from build123d import *

# Parameters (mm, degrees)
SKIZZE1_W                                           = 135.069444444
SKIZZE1_H                                           = 50
AUFSATZ_LINEAR_AUSTRAGEN1_DEPTH                     = 200
STIRNSENKUNG_F_R_M8_SENKSCHRAUBE_KOPF_B_D           = 9
STIRNSENKUNG_F_R_M8_SENKSCHRAUBE_KOPF_B_CBORE_D     = 15
STIRNSENKUNG_F_R_M8_SENKSCHRAUBE_KOPF_B_CBORE_DEPTH = 34.5
STIRNSENKUNG_F_R_M8_SENKSCHRAUBE_KO_2_D             = 9
STIRNSENKUNG_F_R_M8_SENKSCHRAUBE_KO_2_DEPTH         = 50
STIRNSENKUNG_F_R_M8_SENKSCHRAUBE_KO_2_CBORE_D       = 15
STIRNSENKUNG_F_R_M8_SENKSCHRAUBE_KO_2_CBORE_DEPTH   = 6.5


with BuildPart() as part:
    # Skizze1 → Aufsatz-Linear austragen1 (new body)
    with BuildSketch(Plane.XY):
        Rectangle(SKIZZE1_W, SKIZZE1_H)
    extrude(amount=AUFSATZ_LINEAR_AUSTRAGEN1_DEPTH)

    # Stirnsenkung f_r M8 Senkschraube _Kopf B (through all)
    with Locations(Plane(origin=(0, 25, 0), x_dir=(1, 0, 0), z_dir=(0, 1, 0))):
        with Locations((0, -150)):
            stirnsenkung_f_r_m8_senkschraube_kopf_b = CounterBoreHole(STIRNSENKUNG_F_R_M8_SENKSCHRAUBE_KOPF_B_D / 2, STIRNSENKUNG_F_R_M8_SENKSCHRAUBE_KOPF_B_CBORE_D / 2, STIRNSENKUNG_F_R_M8_SENKSCHRAUBE_KOPF_B_CBORE_DEPTH)

    # Stirnsenkung f_r M8 Senkschraube _Ko 2
    with Locations(Plane(origin=(0, -25, 0), x_dir=(-1, 0, 0), z_dir=(0, -1, 0))):
        with Locations((0, -150)):
            stirnsenkung_f_r_m8_senkschraube_ko_2 = CounterBoreHole(STIRNSENKUNG_F_R_M8_SENKSCHRAUBE_KO_2_D / 2, STIRNSENKUNG_F_R_M8_SENKSCHRAUBE_KO_2_CBORE_D / 2, STIRNSENKUNG_F_R_M8_SENKSCHRAUBE_KO_2_CBORE_DEPTH, depth=STIRNSENKUNG_F_R_M8_SENKSCHRAUBE_KO_2_DEPTH)

    # Spiegeln1: Stirnsenkung f_r M8 Senkschraube _Kopf B, Stirnsenkung f_r M8 Senkschraube _Ko 2 across plane
    add(stirnsenkung_f_r_m8_senkschraube_kopf_b.mirror(Plane.XY.offset(100)), mode=Mode.SUBTRACT)
    add(stirnsenkung_f_r_m8_senkschraube_ko_2.mirror(Plane.XY.offset(100)), mode=Mode.SUBTRACT)

    # Skizze10 → Kernloch für M8 Helicoil1 (revolve, cut)
    with BuildSketch(Plane(origin=(-52.534722222, 25, 185), x_dir=(0, 0, 1), z_dir=(1, 0, 0))):
        Polygon((0, 0), (0, 32.493571569), (4.15, 30), (4.15, 0), align=None)
    kernloch_f_r_m8_helicoil1 = revolve(axis=Axis((-52.534722222, 31.35, 185), (0, -1, 0)), mode=Mode.SUBTRACT)

    # Spiegeln2: Kernloch für M8 Helicoil1 across plane
    add(kernloch_f_r_m8_helicoil1.mirror(Plane(origin=(0, 0, 0), x_dir=(0, 0, 1), z_dir=(1, 0, 0))), mode=Mode.SUBTRACT)

    # Spiegeln3: Kernloch für M8 Helicoil1 across plane
    add(kernloch_f_r_m8_helicoil1.mirror(Plane.XY.offset(100)), mode=Mode.SUBTRACT)

    # Spiegeln3 copy 1 sketch → Spiegeln3 copy 1 (revolve, cut)
    with BuildSketch(Plane(origin=(52.534722222, 25, 15), x_dir=(0, 0, -1), z_dir=(-1, 0, 0))):
        Polygon((0, 0), (0, 32.493571569), (4.15, 30), (4.15, 0), align=None)
    revolve(axis=Axis((52.534722222, 31.35, 15), (0, -1, 0)), mode=Mode.SUBTRACT)


solid = part.part
Model file for the job. Use its own axes, mm. A direction names the side the tool comes from. Coordinates: 2 decimals unless noted, no trailing zeros. Order: outer loops, then holes, each group sorted by start corner. A loop starts at its lowest first (then second) coordinate and runs counter-clockwise, first axis right, second up. Notation, with made-up numbers: (53, 69) -> (102, 69) arc R22 ccw to (102, 89) -> close; hole circle Ø8 at (85.5, 3). An arc over 180 degrees is marked (long way). Return JSON: item names as keys, results as strings. Group by question number.
Item 1: Saw through at B-B on z = 150. Write the cut outline in (x, y).
Item 2: Saw through at C-C on y = 0.5. Write the cut outline in (x, z).
Item 3: Pull direction Z, two halves, no side cores. Call faces 4 (the flat face through (-1, 0, 0)), 5 (the cylindrical face through (0.98, -14.06, 154.39)), 6 (the cylindrical face through (50.01, 10.21, 181.707)), 7 (the flat face through (-1, 0, 200)): pulls with the +Z half, pulls with the -Z half, needs draft (parallel to the pull), parting line crosses it, or undercut.
Item 4: Wall check: line 1 along X through (y, z) = (3.5, 185); line 2 along Z through (x, y) = (0, 12); line 3 along Z through (x, y) = (0, -15.75). Give the ranges that are in metal, low to high. Write a range as [from, to].
Item 5: Tool access for faces 1 (the cylindrical face through (0.976, -21.796, 57.436)), 2 (the flat face through (-1, -25, 99)), 3 (the cylindrical face through (48.483, 10.21, 15.9)): list every direction of +Z, -Z, +X, -X, +Y, -Y with a clear straight run to the whole face (end or side of a thin tool).
Item 6: Flat gauge pins, fed straight in: P1, Ø2, axis at x = 30, y = -13, coming from the -Z side; P2, Ø4.5, axis at x = 2, z = 148.5, coming from the +Y side; P3, Ø7.5, axis at x = 52.53, z = 185, coming from the +Y side; P4, Ø5, axis at x = 52.53, z = 15, coming from the +Y side. Where does each tip first touch, or does it go through?
Item 7: Saw through at A-A on x = 0. Write the cut outline in (y, z), then the cut area to 3 significant figures.
Values found:
{
 "1": {"outline": "(-67.53, -25) -> (-7.5, -25) -> (-7.5, -18.5) -> (-4.5, -18.5) -> (-4.5, -9.5) -> (-7.5, -9.5) -> (-7.5, 25) -> (-67.53, 25) -> close; (4.5, -18.5) -> (7.5, -18.5) -> (7.5, -25) -> (67.53, -25) -> (67.53, 25) -> (7.5, 25) -> (7.5, -9.5) -> (4.5, -9.5) -> close"},
 "2": {"outline": "(-67.53, 0) -> (67.53, 0) -> (67.53, 200) -> (-67.53, 200) -> close; hole circle Ø8.3 at (-52.53, 15); hole circle Ø8.3 at (-52.53, 185); hole circle Ø15 at (0, 50); hole circle Ø15 at (0, 150); hole circle Ø8.3 at (52.53, 15); hole circle Ø8.3 at (52.53, 185)"},
 "3": {"face 4": "pulls with the -Z half", "face 5": "undercut", "face 6": "undercut", "face 7": "pulls with the +Z half"},
 "4": {"line 1": "x = [-67.53, -56.68], [-48.38, 48.38], [56.68, 67.53]", "line 2": "z = [0, 42.5], [57.5, 142.5], [157.5, 200]", "line 3": "z = [0, 45.5], [54.5, 145.5], [154.5, 200]"},
 "5": {"face 1": "-Y", "face 2": "+Z, -Z, +X, -X, -Y", "face 3": "+Y"},
 "6": {"P1": "stops at z = 0", "P2": "stops at y = -9.5", "P3": "stops at y = -5.24", "P4": "stops at y = -5.99"},
 "7": {"outline": "(-25, 0) -> (25, 0) -> (25, 42.5) -> (-9.5, 42.5) -> (-9.5, 45.5) -> (-18.5, 45.5) -> (-18.5, 42.5) -> (-25, 42.5) -> close; (-25, 57.5) -> (-18.5, 57.5) -> (-18.5, 54.5) -> (-9.5, 54.5) -> (-9.5, 57.5) -> (25, 57.5) -> (25, 142.5) -> (-9.5, 142.5) -> (-9.5, 145.5) -> (-18.5, 145.5) -> (-18.5, 142.5) -> (-25, 142.5) -> close; (-25, 157.5) -> (-18.5, 157.5) -> (-18.5, 154.5) -> (-9.5, 154.5) -> (-9.5, 157.5) -> (25, 157.5) -> (25, 200) -> (-25, 200) -> close", "area": "8,610 mm2"}
}
